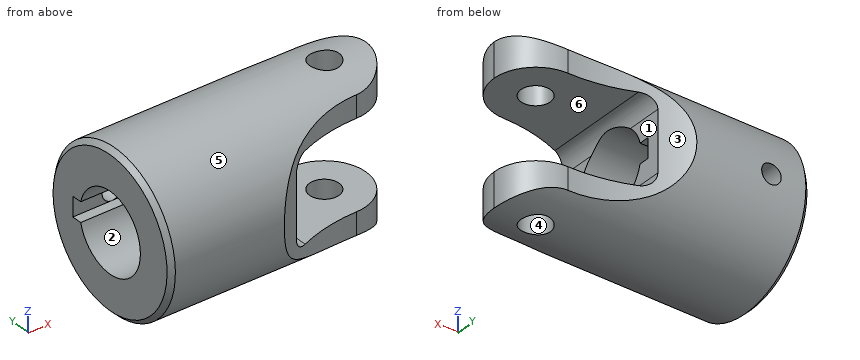
from build123d import *

# Parameters (mm, degrees)
SKETCH1_R               = 25.4
BOSS_EXTRUDE1_DEPTH     = 83.08975
CUT_EXTRUDE1_DEPTH      = 43.688
SKETCH5_R               = 4.76885
CUT_EXTRUDE2_DEPTH      = 43.688
SKETCH6_W               = 13.49375
SKETCH6_H               = 14.29385
CUT_EXTRUDE3_DEPTH      = 43.688
CUT_EXTRUDE4_DEPTH      = 87.376
CUT_EXTRUDE4_DEPTH_BACK = 58.744653114
CHAMFER1_SIZE           = 1.524
SKETCH9_R               = 3.175
CUT_EXTRUDE5_DEPTH      = 91.521967399


with BuildPart() as part:
    # Sketch1 → Boss-Extrude1 (new body)
    with BuildSketch(Plane(origin=(0, 0, 0), x_dir=(0, 0, -1), z_dir=(1, 0, 0))):
        Circle(SKETCH1_R)
    extrude(amount=BOSS_EXTRUDE1_DEPTH)

    # Sketch4 → Cut-Extrude1 (cut, symmetric)
    with BuildSketch(Plane.XY):
        with BuildLine():
            ThreePointArc((69.596, 13.49375), (79.137522129, 9.541522129), (83.08975, 0))
            Line((83.08975, 0), (83.08975, 25.4))
            Line((83.08975, 25.4), (36.9170127, 25.4))
            ThreePointArc((36.9170127, 25.4), (52.205808799, 16.563033999), (69.596, 13.49375))
        make_face()
        with BuildLine():
            Line((36.9170127, -25.4), (83.08975, -25.4))
            Line((83.08975, -25.4), (83.08975, 0))
            ThreePointArc((83.08975, 0), (79.137522129, -9.541522129), (69.596, -13.49375))
            ThreePointArc((69.596, -13.49375), (52.205808799, -16.563033999), (36.9170127, -25.4))
        make_face()
    extrude(amount=CUT_EXTRUDE1_DEPTH, both=True, mode=Mode.SUBTRACT)

    # Sketch5 → Cut-Extrude2 (cut, symmetric)
    with BuildSketch(Plane.XY):
        with Locations((69.596, 0)):
            Circle(SKETCH5_R)
    extrude(amount=CUT_EXTRUDE2_DEPTH, both=True, mode=Mode.SUBTRACT)

    # Sketch6 → Cut-Extrude3 (cut, symmetric)
    with BuildSketch(Plane(origin=(0, 0, 0), x_dir=(1, 0, 0), z_dir=(0, 1, 0))):
        with BuildLine():
            Line((69.596, 0), (69.596, 14.29385))
            Line((69.596, 14.29385), (49.784, 14.29385))
            ThreePointArc((49.784, 14.29385), (46.551107796, 12.954742204), (45.212, 9.72185))
            Line((45.212, 9.72185), (45.212, 0))
            Line((45.212, 0), (69.596, 0))
        make_face()
        with BuildLine():
            Line((69.596, -14.29385), (69.596, 0))
            Line((69.596, 0), (45.212, 0))
            Line((45.212, 0), (45.212, -9.72185))
            ThreePointArc((45.212, -9.72185), (46.551107796, -12.954742204), (49.784, -14.29385))
            Line((49.784, -14.29385), (69.596, -14.29385))
        make_face()
        with Locations((76.342875, -7.146925)):
            Rectangle(SKETCH6_W, SKETCH6_H)
        with Locations((76.342875, 7.146925)):
            Rectangle(SKETCH6_W, SKETCH6_H)
    extrude(amount=CUT_EXTRUDE3_DEPTH, both=True, mode=Mode.SUBTRACT)

    # Sketch7 → Cut-Extrude4 (cut, two sides: drawn at the far end of the back side and taken through both)
    with BuildSketch(Plane(origin=(45.212, 0, 0), x_dir=(0, 0, -1), z_dir=(1, 0, 0)).offset(-CUT_EXTRUDE4_DEPTH_BACK)):
        with BuildLine():
            Line((-3.175, 12.296722124), (-3.175, 15.5956))
            Line((-3.175, 15.5956), (3.175, 15.5956))
            Line((3.175, 15.5956), (3.175, 12.296722124))
            ThreePointArc((3.175, 12.296722124), (0, -12.7), (-3.175, 12.296722124))
        make_face()
    extrude(amount=CUT_EXTRUDE4_DEPTH + CUT_EXTRUDE4_DEPTH_BACK, mode=Mode.SUBTRACT)

    # Chamfer1
    chamfer1_edges = [part.edges().sort_by_distance(p)[0] for p in [
        (0, 0, 25.4),
    ]]
    chamfer(chamfer1_edges, length=CHAMFER1_SIZE)

    # Sketch9 → Cut-Extrude5 (cut, through all)
    with BuildSketch(Plane(origin=(0, 0, 0), x_dir=(1, 0, 0), z_dir=(0, 1, 0))):
        with Locations(Location((12.7, 0, 0), (0, 0, 90))):
            Circle(SKETCH9_R)
    extrude(amount=CUT_EXTRUDE5_DEPTH, mode=Mode.SUBTRACT)


solid = part.part
Verification items for the finished model (mm, model axes). Face numbers are marked on the shaded views. A direction names the side the tool comes from. Give positions to 0.01 mm unless a question says otherwise; leave off trailing zeros. Loops run counter-clockwise (first coordinate to the right, second up) from the corner with the lowest first, then second, coordinate; pieces in that order, holes last.
1. Cross-section at A-A on x = 24.5. Record the cut outline in (y, z) (3 decimals), and give its area (3 significant figures).
Derived:
outline: circle Ø50.8 at (0, 0); hole (12.297, -3.175) - (15.596, -3.175) - (15.596, 3.175) - (12.297, 3.175) arc R12.7 ccw (long way) to start
area: 1,500 mm2
2. Cross-section at C-C on y = 1. Count the separate pieces of the cut face and the enclosed holes in it, and give its area (3 significant figures).
Derived:
separate pieces: 4
enclosed holes: 0
area: 1,790 mm2
3. Release check for a two-part mould opening along Y. For the marked faces 1, 2, 3 and 4 record: +Y half, -Y half, draft (parallel to the pull), parting line (faces both ways), or undercut.
Derived:
face 1: draft
face 2: undercut
face 3: +Y half
face 4: undercut
4. Cross-section at B-B on x = 57. Record the cut outline in (y, z).
Derived:
outline: (-15.08, -20.44) arc R25.4 ccw to (15.08, -20.44) - (15.08, -14.29) - (-15.08, -14.29) - close; (-15.08, 14.29) - (15.08, 14.29) - (15.08, 20.44) arc R25.4 ccw to (-15.08, 20.44) - close
5. Material ranges on probe 1 along Y at (x, z) = (31, 0); probe 2 along Y at (x, z) = (70, 20); probe 3 along Z at (x, y) = (28, 6.5), recorded low to high.
Derived:
probe 1: y = -25.4 to -12.7, 15.6 to 25.4
probe 2: y = -13.49 to -4.75, 4.75 to 13.49
probe 3: z = -24.55 to -10.91, 10.91 to 24.55
6. Tool access check on the marked faces 5 and 6. Record the directions out of +Z, -Z, +X, -X, +Y, -Y that give a thin tool (end or side, any length) a straight path to the whole face; none if there is none.
Derived:
face 5: +X, -X
face 6: +X, +Y, -Y
7. Cross-section at D-D on x = 42. Record the cut outline in (y, z) (3 decimals), and give its area (3 significant figures).
Derived:
outline: (-21.643, -13.295) arc R25.4 ccw to (21.643, -13.295) - (21.643, 13.295) arc R25.4 ccw to (-21.643, 13.295) - close; hole (12.297, -3.175) - (15.596, -3.175) - (15.596, 3.175) - (12.297, 3.175) arc R12.7 ccw (long way) to start
area: 1,370 mm2
8. Go/stop test with flat-tipped pins: P1, Ø12.5, axis at y = -14, z = -1, coming from the +X side; P2, Ø3, axis at x = 19, y = -17.5, coming from the -Z side; P3, Ø5, axis at x = 6.5, z = 1, coming from the -Y side. Record where each tip stops, or that it passes through.
Derived:
P1: stops at x = 45.21
P2: stops at z = -19.73
P3: stops at y = -25.4
